Can you work these out from the drawing? Everything is in mm from the part's minimum corner. A direction names the side the tool comes from. Round coordinates to 2 decimals unless told otherwise and drop trailing zeros. Order: outer loops, then holes, each group sorted by start corner. A loop starts at its lowest first (then second) coordinate and runs counter-clockwise, first axis right, second up. Notation, with made-up numbers: M 63,86.25 L 72,86.25 A15 cw 72,102.25 Z; hole C 21.25,54 d2. An arc over 180 degrees is marked long. Write item = value, one per line. Start each with the question number.
Item 1: We'd pull the mould along X, two halves only. Please class the marked faces 1, 2 and 3: pulls with the +X half, pulls with the -X half, needs draft (parallel to the pull), parting line crosses it, or undercut.
Item 2: I want a section at A-A, the plane z = 33. List the corners of the cut face in (x, y) for me, plus the area to 3 significant figures.
Item 3: I want a section at B-B, the plane y = 28. List the corners of the cut face in (x, z) for me, plus the area to 3 significant figures.
Item 4: I want a section at D-D, the plane x = 35. List the corners of the cut face in (y, z) for me.
Item 5: I'm going to push flat-ended pins straight in: P1, Ø4, axis at x = 20, y = 21, coming from the +Z side; P2, Ø5, axis at x = 8, y = 7.5, coming from the +Z side; P3, Ø1, axis at x = 6, z = 19.5, coming from the -Y side. Where does each tip first touch, or does it pass through?
Item 6: I want a section at C-C, the plane x = 47.5. List the corners of the cut face in (y, z) for me.
Item 7: Please list where these lines run through material, in increasing order: L1, parallel to Z at x = 34.5, y = 29; L2, parallel to Y at x = 3, z = 29; L3, parallel to Z at x = 24, y = 7.
Item 8: For the marked faces 4 and 5, which set-ups out of +Z, -Z, +X, -X, +Y, -Y let a thin tool reach every point of the face, with its end or its side?
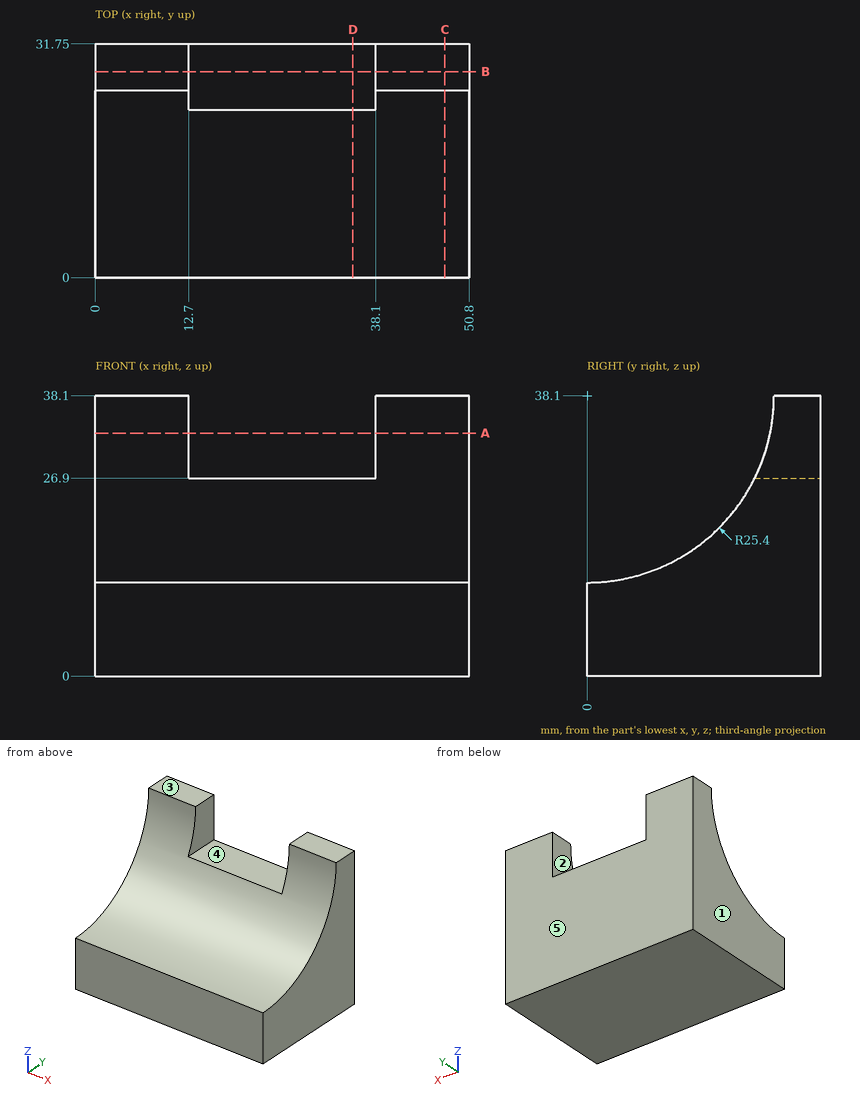
Filled in:
q1.face_1 = pulls with the -X half
q1.face_2 = undercut
q1.face_3 = needs draft
q2.outline = M 0,24.88 L 12.7,24.88 L 12.7,31.75 L 0,31.75 Z; M 38.1,24.88 L 50.8,24.88 L 50.8,31.75 L 38.1,31.75 Z
q2.area = 174 mm^2
q3.outline = M 0,0 L 50.8,0 L 50.8,38.1 L 38.1,38.1 L 38.1,26.9 L 12.7,26.9 L 12.7,38.1 L 0,38.1 Z
q3.area = 1,650 mm^2
q4.outline = M 0,0 L 31.75,0 L 31.75,26.9 L 22.8,26.9 A25.4 cw 0,12.7 Z
q5.P1 = 26.9
q5.P2 = 14.75
q5.P3 = 16.74
q6.outline = M 0,0 L 31.75,0 L 31.75,38.1 L 25.4,38.1 A25.4 cw 0,12.7 Z
q7.L1 = 0 to 26.9
q7.L2 = 23.71 to 31.75
q7.L3 = 0 to 13.68
q8.face_4 = +Z, +Y, -Y
q8.face_5 = +Z, -Z, +X, -X, +Y
